```python
from build123d import *

# Parameters (mm, degrees)
SKETCH_1_R      = 3
EXTRUDE_1_DEPTH = 10


with BuildPart() as part:
    # Эскиз1 → Бобышка-Вытянуть1 (new body)
    with BuildSketch(Plane(origin=(0, 0, 0), x_dir=(1, 0, 0), z_dir=(0, 1, 0))):
        with BuildLine():
            ThreePointArc((-7.075672476, -38.267057593), (0, -50), (7.075672476, -38.267057593))
            ThreePointArc((7.075672476, -38.267057593), (5.504494197, -34.399886744), (4.729224066, -30.298354373))
            Line((4.729224066, -30.298354373), (3.594110581, -17.323947875))
            ThreePointArc((3.594110581, -17.323947875), (4.107078394, -10.538940279), (6.762537722, -4.27411787))
            ThreePointArc((6.762537722, -4.27411787), (0, 8), (-6.762537722, -4.27411787))
            ThreePointArc((-6.762537722, -4.27411787), (-4.107078394, -10.538940279), (-3.594110581, -17.323947875))
            Line((-3.594110581, -17.323947875), (-4.729224066, -30.298354373))
            ThreePointArc((-4.729224066, -30.298354373), (-5.504494197, -34.399886744), (-7.075672476, -38.267057593))
        make_face()
        with Locations((0, -42)):
            Circle(SKETCH_1_R, mode=Mode.SUBTRACT)
        Circle(SKETCH_1_R, mode=Mode.SUBTRACT)
    extrude(amount=EXTRUDE_1_DEPTH)


solid = part.part
```
Geometry check sheet. Reference: the model listing, model coordinates, mm. A direction names the side the tool comes from. Round coordinates to 2 decimals unless told otherwise and drop trailing zeros. Order: outer loops, then holes, each group sorted by start corner. A loop starts at its lowest first (then second) coordinate and runs counter-clockwise, first axis right, second up. Notation, with made-up numbers: (-1, 74.5) -> (36, 74.5) arc R34 ccw to (36, 108.5) -> close; hole circle Ø9 at (-31, 37). An arc over 180 degrees is marked (long way). Return JSON: item names as keys, results as strings. Group by question number.
Q1. Gauge pin test, flat ends, axial feed: pin 1 (6 mm diameter, centred on x = -6, y = 5.5, fed in from -Z); pin 2 (6 mm diameter, centred on y = 1.5, z = 20, fed in from +X); pin 3 (2 mm diameter, centred on y = 9, z = 4, fed in from +X). Record the tip position at first contact, or that the pin passes through.
Q2. Material ranges on probe 1 along X at (y, z) = (7.75, 0); probe 2 along Z at (x, y) = (-1.25, 2.75); probe 3 along Z at (x, y) = (0, 7), recorded low to high. Write a range as from..to.
Q3. Section check A-A, the plane z = 0. Record the boundary of the cut face in (x, y).
Q4. Section check D-D, the plane x = -5.5. Record the boundary of the cut face in (y, z), plus the area to 3 significant figures.
Q5. Section check C-C, the plane y = 6.25. Record the boundary of the cut face in (x, z).
Q6. Tool access check on faces 1 (the flat face through (-4.154, 4.93, 23.72)), 2 (the flat face through (0, 0, 21)), 3 (the cylindrical face through (5.521, 4.93, 34.456)). Record the directions out of +Z, -Z, +X, -X, +Y, -Y that give a thin tool (end or side, any length) a straight path to the whole face; none if there is none.
Q7. Release check for a two-part mould opening along X. For faces 4 (the cylindrical face through (0, 5, 39)), 5 (the cylindrical face through (4, 5, 11)), 6 (the cylindrical face through (0, 5, 50)), 7 (the cylindrical face through (-3, 5, 0)) record: released by +X, released by -X, zero draft, split by the parting line, or undercut.
Q8. Section check B-B, the plane x = 0. Record the boundary of the cut face in (y, z), plus the area to 3 significant figures.
Numbers:
{
 "1": {"pin 1": "z = -7.42", "pin 2": "x = 4.09", "pin 3": "x = 7.42"},
 "2": {"probe 1": "-8..-3, 3..8", "probe 2": "-7.9..-2.73, 2.73..39.27, 44.73..49.9", "probe 3": "-8..-3, 3..39, 45..50"},
 "3": {"outline": "(-8, 0) -> (-3, 0) -> (-3, 10) -> (-8, 10) -> close; (3, 0) -> (8, 0) -> (8, 10) -> (3, 10) -> close"},
 "4": {"outline": "(0, -5.81) -> (10, -5.81) -> (10, 6.58) -> (0, 6.58) -> close; (0, 34.38) -> (10, 34.38) -> (10, 47.81) -> (0, 47.81) -> close", "area": "258 mm^2"},
 "5": {"outline": "(-7.08, 38.27) arc R21 cw to (-4.73, 30.3) -> (-3.59, 17.32) arc R21 cw to (-6.76, 4.27) arc R8 ccw (long way) to (6.76, 4.27) arc R21 cw to (3.59, 17.32) -> (4.73, 30.3) arc R21 cw to (7.08, 38.27) arc R8 ccw (long way) to start; hole circle Ø6 at (0, 0); hole circle Ø6 at (0, 42)"},
 "6": {"face 1": "-X, +Y, -Y", "face 2": "+Z, -Z, +X, -X, -Y", "face 3": "+X, +Y, -Y"},
 "7": {"face 4": "undercut", "face 5": "released by +X", "face 6": "split by the parting line", "face 7": "undercut"},
 "8": {"outline": "(0, -8) -> (10, -8) -> (10, -3) -> (0, -3) -> close; (0, 3) -> (10, 3) -> (10, 39) -> (0, 39) -> close; (0, 45) -> (10, 45) -> (10, 50) -> (0, 50) -> close", "area": "460 mm^2"}
}
